from build123d import *
from build123d import SkipClean  # not in build123d's __all__

# Parameters (mm, degrees)
F1_DEPTH = 7.62
F2_DEPTH = 7.62
F0_W     = 2.54
F0_H     = 5.08
F3_DEPTH = 7.62
F5_DEPTH = 2.54
F6_DEPTH = 36.831


# Not quite as in the source:
# - a feature names something its author has since deleted; it is built from what else it names


with BuildPart() as f1:
    # F0 (on Front) → F1 (new body)
    with BuildSketch(Plane.XZ):
        Polygon((8.89, 0), (0, 0), (-8.89, 0), (-11.43, 0), (-25.4, 0), (-25.4, -5.08), (25.4, -5.08), (25.4, 0), (11.43, 0), align=None)
    extrude(amount=F1_DEPTH)

    # F0 (on Front) → F2 (join)
    with BuildSketch(Plane.XZ):
        Polygon((8.89, 0), (0, 0), (-8.89, 0), (-11.43, 0), (-25.4, 0), (-25.4, -5.08), (25.4, -5.08), (25.4, 0), (11.43, 0), align=None)
    extrude(amount=F2_DEPTH)

    # F0 (on Front) → F3 (join)
    with BuildSketch(Plane.XZ):
        with Locations((-10.16, 2.54)):
            Rectangle(F0_W, F0_H)
        with Locations((10.16, 2.54)):
            Rectangle(F0_W, F0_H)
    extrude(amount=F3_DEPTH)

    # F4 (on face) → F5 (join)
    with BuildSketch(Plane(origin=(-11.43, 0, 0), x_dir=(0, -1, 0), z_dir=(-1, 0, 0))):
        with BuildLine():
            Line((6.1004036929, 5.08), (7.62, 5.08))
            ThreePointArc((7.62, 5.08), (3.81, 7.8260926284), (0, 5.08))
            Line((0, 5.08), (1.5195963071, 5.08))
            ThreePointArc((1.5195963071, 5.08), (3.81, 6.5219786325), (6.1004036929, 5.08))
        make_face()
    extrude(amount=-F5_DEPTH)

    # F4 (on face) → F6 (cut, through all)
    with BuildSketch(Plane(origin=(-11.43, 0, 0), x_dir=(0, -1, 0), z_dir=(-1, 0, 0))):
        with BuildLine():
            ThreePointArc((6.35, 3.9819786325), (6.2868150294, 4.5449948934), (6.1004036929, 5.08))
            Line((6.1004036929, 5.08), (1.5195963071, 5.08))
            ThreePointArc((1.5195963071, 5.08), (3.2469837391, 1.5051636031), (6.35, 3.9819786325))
        make_face()
    with SkipClean():  # cleaning this boolean's faces spoils the solid; the shape is the same uncleaned
        extrude(amount=-F6_DEPTH, mode=Mode.SUBTRACT)

    # F7: F1 across plane


with BuildPart() as f1_1:
    add(f1.part, clean=False)
    with SkipClean():  # cleaning this boolean's faces spoils the solid; the shape is the same uncleaned
        add(f1.part.mirror(Plane.YZ), clean=False)


solid = f1_1.part
The listing builds one solid part. Answer for the finished solid, in the listing's coordinates (mm). A direction names the side the tool comes from. Give positions to 0.01 mm unless a question says otherwise; leave off trailing zeros. Order: outer loops, then holes, each group sorted by start corner. A loop starts at its lowest first (then second) coordinate and runs counter-clockwise, first axis right, second up. Notation, with made-up numbers: (-13, 70) - (43, 70) arc R22 cw to (43, 83) - close; hole circle Ø5 at (-7, 17.5). An arc over 180 degrees is marked (long way). Answer as CSV lines item,"result".
Q1. Each of these flat-tipped pins is pushed along its axis until it touches: pin 1 Ø4 at (y, z) = (-5.5, 6) entering from +X; pin 2 Ø4 at (x, y) = (1.5, -4) entering from +Z. Where does it stop, or does it pass through?
Answer key:
pin 1,"stops at x = 11.43"
pin 2,"stops at z = 0"
Q2. Which of the six approach directions +Z, -Z, +X, -X, +Y, -Y give full straight-line access (tool end or side, diameter ignored) to faces 1 (the face through (0, -4, -5.08)), 2 (the face through (0, -7.62, -2)), 3 (the face through (-18, -4, 0)), 4 (the face through (19, -4, 0)), 5 (the face through (8.89, -4, 1))?
Answer key:
face 1,"-Z, +X, -X, +Y, -Y"
face 2,"+Z, -Z, +X, -X, -Y"
face 3,"+Z, -X, +Y, -Y"
face 4,"+Z, +X, +Y, -Y"
face 5,"+Z, +Y, -Y"
Q3. Determine the mould class of faces 6 (the face through (-10.178, -3.88, 7.825)), 7 (the face through (-8.89, -4, 1)), 8 (the face through (25.4, -4, -3)), 9 (the face through (-11.43, -4, 1)) for opening direction X: pulls with the +X half, pulls with the -X half, needs draft (parallel to the pull), parting line crosses it, or undercut.
Answer key:
face 6,"needs draft"
face 7,"undercut"
face 8,"pulls with the +X half"
face 9,"pulls with the -X half"
Q4. A cutting plane is placed at B-B, the plane z = 1. Determine the outline of the cut face in (x, y).
Answer key:
outline,"(-11.43, -7.62) - (-8.89, -7.62) - (-8.89, 0) - (-11.43, 0) - close; (8.89, -7.62) - (11.43, -7.62) - (11.43, 0) - (8.89, 0) - close"
Q5. Straight lines are drawn through the part: L1, parallel to X at y = -1, z = 3; L2, parallel to Z at x = 15.5, y = -5.5. For each, find the intervals that lie inside material, in ascending order.
Answer key:
L1,"x = -11.43 to -8.89, 8.89 to 11.43"
L2,"z = -5.08 to 0"
Q6. A cutting plane is placed at A-A, the plane y = -3.81. Determine the outline of the cut face in (x, z).
Answer key:
outline,"(-25.4, -5.08) - (25.4, -5.08) - (25.4, 0) - (11.43, 0) - (11.43, 1.44) - (8.89, 1.44) - (8.89, 0) - (-8.89, 0) - (-8.89, 1.44) - (-11.43, 1.44) - (-11.43, 0) - (-25.4, 0) - close; (-11.43, 6.52) - (-8.89, 6.52) - (-8.89, 7.83) - (-11.43, 7.83) - close; (8.89, 6.52) - (11.43, 6.52) - (11.43, 7.83) - (8.89, 7.83) - close"
Q7. A cutting plane is placed at C-C, the plane x = -1. Determine the outline of the cut face in (y, z).
Answer key:
outline,"(-7.62, -5.08) - (0, -5.08) - (0, 0) - (-7.62, 0) - close"
Q8. A cutting plane is placed at D-D, the plane z = 4.5. Determine the outline of the cut face in (x, y).
Answer key:
outline,"(-11.43, -7.62) - (-8.89, -7.62) - (-8.89, -6.3) - (-11.43, -6.3) - close; (-11.43, -1.32) - (-8.89, -1.32) - (-8.89, 0) - (-11.43, 0) - close; (8.89, -7.62) - (11.43, -7.62) - (11.43, -6.3) - (8.89, -6.3) - close; (8.89, -1.32) - (11.43, -1.32) - (11.43, 0) - (8.89, 0) - close"
